Job drawing, mm, ordinate dimensions from the low corner. One solid piece. A direction names the side the tool comes from. Give positions to 0.01 mm unless a question says otherwise; leave off trailing zeros. Order: outer loops, then holes, each group sorted by start corner. A loop starts at its lowest first (then second) coordinate and runs counter-clockwise, first axis right, second up. Notation, with made-up numbers: M 10,-9.75 L 31,-9.75 A9 cw 31,-2.75 Z; hole C -2.75,20 d11. An arc over 180 degrees is marked long. One line per question, with ' | ' between items.
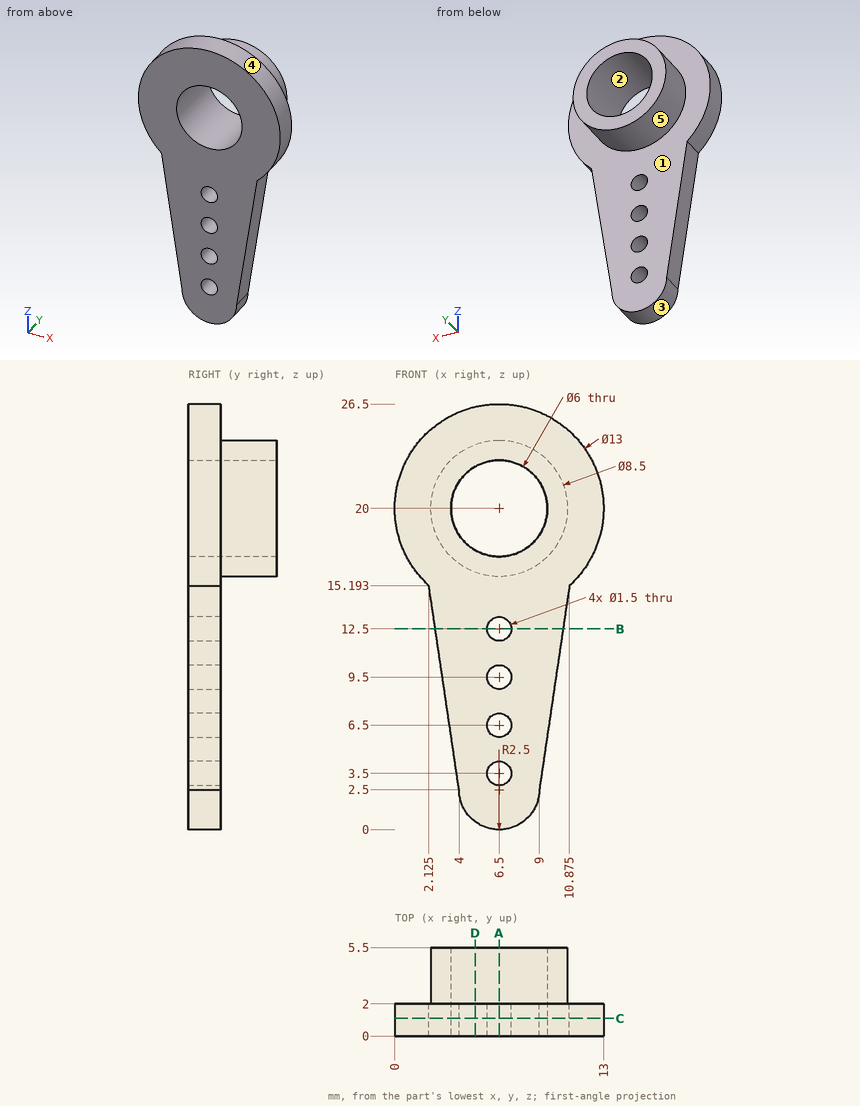
1. Drop flat-ended pins along their axis: pin 1 (2 mm diameter, centred on x = 6.5, z = 6.5, fed in from +Y); pin 2 (1.2 mm diameter, centred on x = 6.5, z = 9.5, fed in from -Y); pin 3 (3 mm diameter, centred on x = 4, z = 17.5, fed in from -Y); pin 4 (1 mm diameter, centred on x = 9, y = 3, fed in from -Z). Give the stop position or say it passes through.
Worked out:
pin 1: stops at y = 2 | pin 2: passes through | pin 3: stops at y = 0 | pin 4: stops at z = 16.25
2. Tool access for the marked faces 4 and 5: list every direction of +Z, -Z, +X, -X, +Y, -Y with a clear straight run to the whole face (end or side of a thin tool).
Worked out:
face 4: +Y, -Y | face 5: +Y
3. Probe L1, parallel to X at y = 1.95, z = 20; L2, parallel to X at y = 1.1, z = 9.5; L3, parallel to Y at x = 1.25, z = 19. List the from-to ranges inside material, lowest first. Write a range as from..to.
Worked out:
L1: x = 0..3.5, 9.5..13 | L2: x = 2.97..5.75, 7.25..10.03 | L3: y = 0..2
4. Slice it at A-A on x = 6.5. Give the cut face in (y, z).
Worked out:
outline: M 0,0 L 2,0 L 2,2.75 L 0,2.75 Z; M 0,4.25 L 2,4.25 L 2,5.75 L 0,5.75 Z; M 0,7.25 L 2,7.25 L 2,8.75 L 0,8.75 Z; M 0,10.25 L 2,10.25 L 2,11.75 L 0,11.75 Z; M 0,13.25 L 2,13.25 L 2,15.75 L 5.5,15.75 L 5.5,17 L 0,17 Z; M 0,23 L 5.5,23 L 5.5,24.25 L 2,24.25 L 2,26.5 L 0,26.5 Z
5. Slice it at B-B on z = 12.5. Give the cut face in (x, y).
Worked out:
outline: M 2.52,0 L 5.75,0 L 5.75,2 L 2.52,2 Z; M 7.25,0 L 10.48,0 L 10.48,2 L 7.25,2 Z
6. Slice it at C-C on y = 1.1. Give the number of separate pieces and of enclosed holes in the cut face, then the cut area to 3 significant figures.
Worked out:
separate pieces: 1 | enclosed holes: 5 | area: 184 mm2
7. Slice it at D-D on x = 5. Give the cut face in (y, z) (1 decimal), then the cut area to 3 significant figures.
Worked out:
outline: M 0,0.5 L 2,0.5 L 2,16 L 5.5,16 L 5.5,17.4 L 0,17.4 Z; M 0,22.6 L 5.5,22.6 L 5.5,24 L 2,24 L 2,26.3 L 0,26.3 Z | area: 50.9 mm2
8. Mould opens along X. For the marked faces 1, 2 and 3 say: released by +X, released by -X, zero draft, split by the parting line, or undercut.
Worked out:
face 1: zero draft | face 2: undercut | face 3: split by the parting line
